Can you work these out from the model? Positions are in its coordinate system, mm. A direction names the side the tool comes from. Give positions to 0.01 mm unless a question says otherwise; leave off trailing zeros. Loops run counter-clockwise (first coordinate to the right, second up) from the corner with the lowest first, then second, coordinate; pieces in that order, holes last. Notation, with made-up numbers: (-35, 89) -> (-6, 89) arc R26 cw to (-6, 118) -> close; hole circle Ø4 at (78, 53). An arc over 180 degrees is marked (long way). One line per question, with ' | ' between items.
from build123d import *

# Parameters (mm, degrees)
SKETCH2_W                    = 9.4996
SKETCH2_H                    = 44.1706
F_3_8_16_TAPPED_HOLE2_REACH  = 91.671
F_3_8_16_TAPPED_HOLE2_BORE_R = 3.96875
CIRPATTERN1_COUNT            = 6
CIRPATTERN2_COUNT            = 6


with BuildPart() as part:
    # Sketch2 → Revolve1 (revolve)
    with BuildSketch(Plane.XY, mode=Mode.PRIVATE) as revolve1_sk:
        with Locations((-30.1498, 22.0853)):
            Rectangle(SKETCH2_W, SKETCH2_H)
    revolve(revolve1_sk.sketch.rotate(Axis((0, 0, 0), (0, 1, 0)), 270), axis=Axis((0, 0, 0), (0, 1, 0)))

    # 3_8-16 Tapped Hole2 bore → 3_8-16 Tapped Hole2 (cut, up to next)
    with BuildSketch(Plane(origin=(34.8996, 0, 0), x_dir=(0, 0, -1), z_dir=(1, 0, 0)), mode=Mode.PRIVATE) as f_3_8_16_tapped_hole2_sk1:
        with Locations((0, 24.4856)):
            Circle(F_3_8_16_TAPPED_HOLE2_BORE_R)
    f_3_8_16_tapped_hole2_tool1 = extrude(f_3_8_16_tapped_hole2_sk1.sketch, amount=-F_3_8_16_TAPPED_HOLE2_REACH, mode=Mode.PRIVATE) & part.part
    f_3_8_16_tapped_hole2 = f_3_8_16_tapped_hole2_tool1.solids().sort_by_distance((34.8996, 24.4856, 0))[0]
    add(f_3_8_16_tapped_hole2, mode=Mode.SUBTRACT)

    # CirPattern1: 3_8-16 Tapped Hole2 ×6 about axis
    cirpattern1_axis = Axis((0, 44.1706, 0), (0, -1, 0))
    for i in range(1, CIRPATTERN1_COUNT):
        add(f_3_8_16_tapped_hole2.rotate(cirpattern1_axis, i * 360 / CIRPATTERN1_COUNT), mode=Mode.SUBTRACT)

    # Sketch14 → Tap Drill for _10-32 Tap1 (revolve, cut)
    with BuildSketch(Plane(origin=(0, 34.036, 34.8996), x_dir=(0, -1, 0), z_dir=(1, 0, 0))):
        Polygon((0, 0), (0, 8.833317848), (2.0193, 7.62), (2.0193, 0), align=None)
    tap_drill_for_10_32_tap1 = revolve(axis=Axis((0, 34.036, 41.2496), (0, 0, -1)), mode=Mode.SUBTRACT)

    # CirPattern2: Tap Drill for _10-32 Tap1 ×6 about axis
    cirpattern2_axis = Axis((0, 0, 0), (0, -1, 0))
    for i in range(1, CIRPATTERN2_COUNT):
        add(tap_drill_for_10_32_tap1.rotate(cirpattern2_axis, i * 360 / CIRPATTERN2_COUNT), mode=Mode.SUBTRACT)


solid = part.part
Q1. On a 3-axis mill with a long thin cutter (end or side, diameter ignored), from which of +Z, -Z, +X, -X, +Y, -Y can I reach the whole of each face in a straight line? I mean faces 1 (the face through (0.134, 33.712, 26.277)), 2 (the face through (-1.79, 33.1, -31.14)), 3 (the face through (-22.824, 33.712, -13.022)). Say none if no direction works.
Entries:
face 1: +Z | face 2: -Z | face 3: none
Q2. If I drill on probe 1 along Y at (x, z) = (0, 30.75); probe 2 along X at (y, z) = (5.5, 1); probe 3 along Y at (x, z) = (31, 0), over which ranges is the centre line in solid material (lowest first)? Write a range as from..to.
Entries:
probe 1: 0..32.02, 36.06..44.17 | probe 2: -34.89..-25.38, 25.38..34.89 | probe 3: 0..20.52, 28.45..44.17
Q3. If we section it at A-A (z = 0): Write out the boundary of the cut face in (x, y), plus the area to 3 significant figures.
Entries:
outline: (-34.9, 0) -> (-25.4, 0) -> (-25.4, 20.52) -> (-34.9, 20.52) -> close; (-34.9, 28.45) -> (-25.4, 28.45) -> (-25.4, 44.17) -> (-34.9, 44.17) -> close; (25.4, 0) -> (34.9, 0) -> (34.9, 20.52) -> (25.4, 20.52) -> close; (25.4, 28.45) -> (34.9, 28.45) -> (34.9, 44.17) -> (25.4, 44.17) -> close | area: 688 mm²
Q4. If we section it at B-B (x = -7): Write out the boundary of the cut face in (y, z), plus the area to 3 significant figures.
Entries:
outline: (0, -34.19) -> (44.17, -34.19) -> (44.17, -24.42) -> (0, -24.42) -> close; (0, 24.42) -> (44.17, 24.42) -> (44.17, 34.19) -> (0, 34.19) -> close | area: 863 mm²
Q5. If we section it at C-C (y = 9): Write out the boundary of the cut face in (x, z).
Entries:
outline: circle Ø69.8 at (0, 0); hole circle Ø50.8 at (0, 0)
Q6. If we mould it in two halves opening along Z, with no side actions, what happens to faces 4 (the face through (-22.69, 33.71, 13.25)), 5 (the face through (-0.134, 33.712, -26.277)), 6 (the face through (1.79, 33.1, 31.14))? For each: pulls with the +Z half, pulls with the -Z half, needs draft (parallel to the pull), parting line crosses it, or undercut.
Entries:
face 4: undercut | face 5: pulls with the -Z half | face 6: needs draft
Q7. For pin 1 Ø5 at (x, y) = (4, 22) entering from -Z; pin 2 Ø10 at (y, z) = (13.5, -25) entering from +X; pin 3 Ø6 at (y, z) = (24.5, -2.5) entering from +X, each with a flat end and sliding along its axis, tell me the tip position at first contact or that it passes through.
Entries:
pin 1: z = -34.87 | pin 2: x = 28.6 | pin 3: x = 34.8
